Here's how the part is built. I have some questions about the finished solid (model axes, mm). Face numbers are marked on the shaded views. Round coordinates to 2 decimals unless told otherwise and drop trailing zeros. Write each loop counter-clockwise with the first axis right and the second up, starting at its lowest first coordinate (ties: lowest second). Pieces come first, ordered by that corner, then holes. Notation, with made-up numbers: (42, 55.5) -> (95, 55.5) arc R30 ccw to (95, 77.5) -> close; hole circle Ø9 at (32, -16.75). An arc over 180 degrees is marked (long way). Put each result on its own line as item: value. Start each with the question number.
1) I want a section at C-C, the plane z = 16. List the corners of the cut face in (x, y) for me, then the cut area to 3 significant figures.
2) I want a section at D-D, the plane y = 3.25. List the corners of the cut face in (x, z) for me.
3) If I drill on line 1 along X through (y, z) = (21.25, -1.5); line 2 along X through (y, z) = (1.55, 0); line 3 along Z through (x, y) = (14.5, 2.25), over which ranges is the centre line in solid material (lowest first)? Write a range as [from, to].
4) I want a section at A-A, the plane y = 19. List the corners of the cut face in (x, z) for me.
5) I want a section at B-B, the plane x = 0. List the corners of the cut face in (y, z) for me, then the cut area to 3 significant figures.
6) Will these pins go through, and if not, where does the flat tip stop? P1, Ø2, axis at x = -5.5, z = 8.5, coming from the +Y side; P2, Ø1.2, axis at x = 5, y = 27, coming from the -Z side; P3, Ø0.6, axis at x = 8, z = 0, coming from the +Y side.
7) We'd pull the mould along X, two halves only. Please class the marked faces 1, 2, 3 and 4: released by +X, released by -X, zero draft, split by the parting line, or undercut.
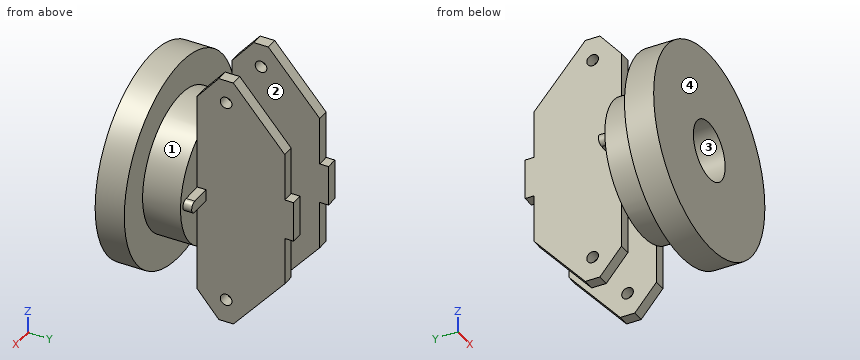
from build123d import *

# Parameters (mm, degrees)
SKETCH1_R           = 17.5
BOSS_EXTRUDE1_DEPTH = 5
SKETCH2_R           = 11.75
BOSS_EXTRUDE2_DEPTH = 6.5
BOSS_EXTRUDE4_DEPTH = 1.5
SKETCH4_R           = 1
BOSS_EXTRUDE5_DEPTH = 2
SKETCH5_R           = 5
CUT_EXTRUDE1_DEPTH  = 5


with BuildPart() as part:
    # Sketch1 → Boss-Extrude1 (new body)
    with BuildSketch(Plane(origin=(0, 0, 0), x_dir=(1, 0, 0), z_dir=(0, 1, 0))):
        with Locations(Location((0, 0, 0), (0, 0, 270))):
            Circle(SKETCH1_R)
    extrude(amount=BOSS_EXTRUDE1_DEPTH)

    # Sketch2 → Boss-Extrude2 (add)
    with BuildSketch(Plane(origin=(0, 5, 0), x_dir=(1, 0, 0), z_dir=(0, 1, 0))):
        with Locations(Location((0, 0, 0), (0, 0, 90))):
            Circle(SKETCH2_R)
    extrude(amount=BOSS_EXTRUDE2_DEPTH)

    # Sketch3 → Boss-Extrude4 (add)
    with BuildSketch(Plane(origin=(0, 11.5, 0), x_dir=(1, 0, 0), z_dir=(0, 1, 0))):
        with BuildLine():
            Line((-6.5, 0), (-6.5, 1))
            Line((-6.5, 1), (-10, 1))
            ThreePointArc((-10, 1), (-11, 0), (-10, -1))
            Line((-10, -1), (-6.5, -1))
            Line((-6.5, -1), (-6.5, 0))
        make_face()
        with BuildLine():
            Line((6.5, -1), (6.5, 0))
            Line((6.5, 0), (6.5, 1))
            Line((6.5, 1), (10, 1))
            ThreePointArc((10, 1), (11, 0), (10, -1))
            Line((10, -1), (6.5, -1))
        make_face()
    extrude(amount=BOSS_EXTRUDE4_DEPTH)

    # Sketch4 → Boss-Extrude5 (add)
    with BuildSketch(Plane(origin=(-6.5, 0, 0), x_dir=(0, 0, -1), z_dir=(1, 0, 0))):
        Polygon((-17.5, 11.5), (17.5, 11.5), (21.904755548, 15.196028756), (21.904755548, 17.696028756), (11.75, 26.5), (3.5, 26.5), (3.5, 28), (-3.5, 28), (-3.5, 26.5), (-11.75, 26.5), (-21.904755548, 17.696028756), (-21.904755548, 15.196028756), align=None)
        with Locations((17.904755548, 16.446028756)):
            Circle(SKETCH4_R, mode=Mode.SUBTRACT)
        with Locations(Location((-17.904755548, 16.446028756, 0), (0, 0, 180))):
            Circle(SKETCH4_R, mode=Mode.SUBTRACT)
    boss_extrude5 = extrude(amount=BOSS_EXTRUDE5_DEPTH)

    # Mirror1: Boss-Extrude5 across plane
    add(boss_extrude5.mirror(Plane(origin=(0, 0, 0), x_dir=(0, 0, 1), z_dir=(1, 0, 0))))

    # Sketch5 → Cut-Extrude1 (cut)
    with BuildSketch(Plane.XZ):
        with Locations(Location((0, 0, 0), (0, 0, 270))):
            Circle(SKETCH5_R)
    extrude(amount=-CUT_EXTRUDE1_DEPTH, mode=Mode.SUBTRACT)


solid = part.part
Findings:
1. outline: (-7.09, 0) -> (7.09, 0) -> (7.09, 5) -> (-7.09, 5) -> close; (-6.5, 11.5) -> (-4.5, 11.5) -> (-4.5, 22.82) -> (-6.5, 22.82) -> close; (4.5, 11.5) -> (6.5, 11.5) -> (6.5, 22.82) -> (4.5, 22.82) -> close
1. area: 116 mm2
2. outline: circle Ø35 at (0, 0); hole circle Ø10 at (0, 0)
3. line 1: x = [-6.5, -4.5], [4.5, 6.5]
3. line 2: x = [-17.5, -5], [5, 17.5]
3. line 3: z = [-9.8, 9.8]
4. outline: (-6.5, -20.4) -> (-4.5, -20.4) -> (-4.5, 20.4) -> (-6.5, 20.4) -> close; (4.5, -20.4) -> (6.5, -20.4) -> (6.5, 20.4) -> (4.5, 20.4) -> close
5. outline: (0, -17.5) -> (5, -17.5) -> (5, -11.75) -> (11.5, -11.75) -> (11.5, 11.75) -> (5, 11.75) -> (5, 17.5) -> (0, 17.5) -> (0, 5) -> (5, 5) -> (5, -5) -> (0, -5) -> close
5. area: 278 mm2
6. P1: stops at y = 26.5
6. P2: stops at z = -11.87
6. P3: stops at y = 13
7. face 1: split by the parting line
7. face 2: undercut
7. face 3: undercut
7. face 4: zero draft
